The listing builds one solid part. Answer for the finished solid, in the listing's coordinates (mm). Face numbers are marked on the shaded views. A direction names the side the tool comes from. Coordinates: 2 decimals unless noted, no trailing zeros. Order: outer loops, then holes, each group sorted by start corner. A loop starts at its lowest first (then second) coordinate and runs counter-clockwise, first axis right, second up.
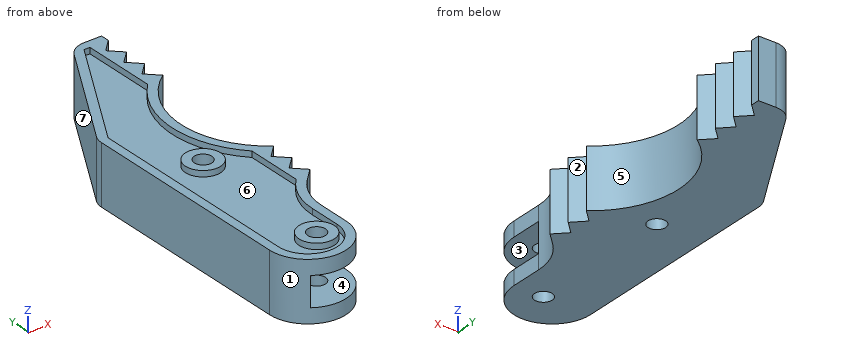
```python
from build123d import *

# Parameters (mm, degrees)
SKETCH1_R           = 1.5
BOSS_EXTRUDE1_DEPTH = 5
CUT_EXTRUDE1_DEPTH  = 2.5
CUT_EXTRUDE2_DEPTH  = 1
SKETCH5_R           = 3
SKETCH5_R_2         = 1.5
EXTRUDE_THIN1_DEPTH = 1
FILLET1_R           = 3.5


with BuildPart() as part:
    # Sketch1 → Boss-Extrude1 (new body, symmetric)
    with BuildSketch(Plane.XY):
        with BuildLine():
            Line((0, 58.5), (-2, 56.5))
            Line((-2, 56.5), (0, 54.5))
            Line((0, 54.5), (-2, 52.5))
            Line((-2, 52.5), (0, 50.5))
            Line((0, 50.5), (-2, 48.5))
            Line((-2, 48.5), (0, 46.5))
            ThreePointArc((0, 46.5), (-6.273030308, 34.3), (0, 22.1))
            Line((0, 22.1), (-2, 20.1))
            Line((-2, 20.1), (0, 18.1))
            Line((0, 18.1), (-2, 16.1))
            Line((-2, 16.1), (0, 14.1))
            Line((0, 14.1), (-2, 12.1))
            ThreePointArc((-2, 12.1), (-4.035298286, 9.053960857), (-4.75, 5.460912703))
            Line((-4.75, 5.460912703), (-4.75, 0))
            ThreePointArc((-4.75, 0), (-11.25, -6.5), (-17.75, 0))
            Line((-17.75, 0), (-17.75, 37.916352203))
            Line((-17.75, 37.916352203), (-5, 60))
            Line((-5, 60), (0, 60))
            Line((0, 60), (0, 58.5))
        make_face()
        with Locations((-9.75, 0)):
            Circle(SKETCH1_R, mode=Mode.SUBTRACT)
        with Locations((-9.75, 25)):
            Circle(SKETCH1_R, mode=Mode.SUBTRACT)
    extrude(amount=BOSS_EXTRUDE1_DEPTH, both=True)

    # Sketch3 → Cut-Extrude1 (cut, symmetric)
    with BuildSketch(Plane.XY):
        with BuildLine():
            Line((-15, -38.410797367), (-15, -6.410797367))
            ThreePointArc((-15, -6.410797367), (-12.082951062, 1.431396204), (-4.75, 5.460912703))
            Line((-4.75, 5.460912703), (-4.75, -38.410797367))
            Line((-4.75, -38.410797367), (-15, -38.410797367))
        make_face()
    extrude(amount=CUT_EXTRUDE1_DEPTH, both=True, mode=Mode.SUBTRACT)

    # Sketch4 → Cut-Extrude2 (cut)
    with BuildSketch(Plane.XY.offset(5)):
        with BuildLine():
            Line((-3.12764747, 58.5), (-4.133974596, 58.5))
            Line((-4.133974596, 58.5), (-16.25, 37.514428415))
            Line((-16.25, 37.514428415), (-16.25, 0))
            ThreePointArc((-16.25, 0), (-11.25, -5), (-6.25, 0))
            Line((-6.25, 0), (-6.25, 5.460912703))
            ThreePointArc((-6.25, 5.460912703), (-5.439227916, 9.583992212), (-3.12764747, 13.093084951))
            Line((-3.12764747, 13.093084951), (-3.12764747, 22.82315148))
            ThreePointArc((-3.12764747, 22.82315148), (-7.773030308, 34.3), (-3.12764747, 45.77684852))
            Line((-3.12764747, 45.77684852), (-3.12764747, 58.5))
        make_face()
    extrude(amount=-CUT_EXTRUDE2_DEPTH, mode=Mode.SUBTRACT)

    # Sketch5 → Extrude-Thin1 (add)
    with BuildSketch(Plane.XY.offset(4)):
        with Locations((-9.75, 0)):
            Circle(SKETCH5_R)
        with Locations((-9.75, 0)):
            Circle(SKETCH5_R_2, mode=Mode.SUBTRACT)
        with Locations((-9.75, 25)):
            Circle(SKETCH5_R)
        with Locations((-9.75, 25)):
            Circle(SKETCH5_R_2, mode=Mode.SUBTRACT)
    extrude(amount=EXTRUDE_THIN1_DEPTH)

    # Fillet1
    fillet1_edges = [part.edges().sort_by_distance(p)[0] for p in [
        (-17.75, 37.916352203, 0),
        (-5, 60, 0),
    ]]
    fillet(fillet1_edges, radius=FILLET1_R)


solid = part.part
```
1) For the marked faces 1, 2 and 3, determine the directions among +Z, -Z, +X, -X, +Y, -Y from which every point of the face is accessible in a straight line to the end or side of a thin tool.
2) A cutting plane is placed at A-A, the plane z = -4.25. Write down the section's boundary in (x, y), plus the area to 3 significant figures.
3) A cutting plane is placed at C-C, the plane y = 25. Write down the section's boundary in (x, z).
4) Each of these flat-tipped pins is pushed along its axis until it touches: P1, Ø4, axis at x = -12.5, z = -3.5, coming from the +Y side; P2, Ø0.8, axis at y = 26.5, z = 4.5, coming from the +X side; P3, Ø1.2, axis at y = 1.5, z = 3.5, coming from the +X side; P4, Ø1.8, axis at x = -9.75, y = 0, coming from the -Z side. Where does it stop, or does it pass through?
5) A cutting plane is placed at B-B, the plane z = 1.25. Write down the section's boundary in (x, y).
6) The mould has two halves that part along X. Classify the marked faces 4, 5, 6 and 7: released by +X, released by -X, zero draft, split by the parting line, or undercut.
7) A cutting plane is placed at D-D, the plane x = -9.5. Count the separate pieces of the cut face and the enclosed holes in it, plus the area to 3 significant figures.
8) Straight lines are drawn through the part: probe 1 along X at (y, z) = (0, 3.1); probe 2 along Y at (x, z) = (-9.75, -3.85); probe 3 along X at (y, z) = (1, 4.5). For each, find the intervals that lie inside material, in ascending order.
Working result:
1. face 1: +Z, -Z, -Y
1. face 2: +Z, -Z, +X
1. face 3: +X, -Y
2. outline: (-17.75, 0) arc R6.5 ccw to (-4.75, 0) - (-4.75, 5.46) arc R9.39 cw to (-2, 12.1) - (0, 14.1) - (-2, 16.1) - (0, 18.1) - (-2, 20.1) - (0, 22.1) arc R15 cw to (0, 46.5) - (-2, 48.5) - (0, 50.5) - (-2, 52.5) - (0, 54.5) - (-2, 56.5) - (0, 58.5) - (0, 60) - (-2.98, 60) arc R3.5 ccw to (-6.01, 58.25) - (-17.28, 38.73) arc R3.5 ccw to (-17.75, 36.98) - close; hole circle Ø3 at (-9.75, 0); hole circle Ø3 at (-9.75, 25)
2. area: 795 mm2
3. outline: (-17.75, -5) - (-11.25, -5) - (-11.25, 5) - (-12.75, 5) - (-12.75, 4) - (-16.25, 4) - (-16.25, 5) - (-17.75, 5) - close; (-8.25, -5) - (-3.04, -5) - (-3.04, 5) - (-4.9, 5) - (-4.9, 4) - (-6.75, 4) - (-6.75, 5) - (-8.25, 5) - close
4. P1: stops at y = 50.47
4. P2: stops at x = -3.83
4. P3: stops at x = -4.75
4. P4: passes through
5. outline: (-17.75, 0) arc R6.5 ccw to (-14.95, -5.34) arc R12 cw to (-4.75, 5.46) arc R9.39 cw to (-2, 12.1) - (0, 14.1) - (-2, 16.1) - (0, 18.1) - (-2, 20.1) - (0, 22.1) arc R15 cw to (0, 46.5) - (-2, 48.5) - (0, 50.5) - (-2, 52.5) - (0, 54.5) - (-2, 56.5) - (0, 58.5) - (0, 60) - (-2.98, 60) arc R3.5 ccw to (-6.01, 58.25) - (-17.28, 38.73) arc R3.5 ccw to (-17.75, 36.98) - close; hole circle Ø3 at (-9.75, 25)
6. face 4: zero draft
6. face 5: released by +X
6. face 6: undercut
6. face 7: released by -X
7. separate pieces: 4
7. enclosed holes: 0
7. area: 449 mm2
8. probe 1: x = -17.75 to -11.25, -8.25 to -4.75
8. probe 2: y = -6.32 to -1.5, 1.5 to 23.5, 26.5 to 51.77
8. probe 3: x = -17.75 to -16.25, -12.58 to -10.87, -8.63 to -6.92, -6.25 to -4.75
